Autodesk Inventor part; units mm, degrees
ref_plane "YZ Plane" through (0, 0, 0) normal (1, 0, 0) x (0, 1, 0)
ref_plane "XZ Plane" through (0, 0, 0) normal (0, 1, 0) x (-1, 0, 0)
ref_plane "XY Plane" through (0, 0, 0) normal (0, 0, 1) x (1, 0, 0)
sketch "Sketch1" plane through (0, 0, 0) normal (0, 0, 1) x (1, 0, 0)
  line L0 (0, 0) -> (34, 0)
  line L1 (34, 0) -> (34, 40)
  line L2 (34, 40) -> (0, 40)
  line L3 (0, 40) -> (0, 0)
  line L4 (-10, 30) -> (0, 30)
  line L5 (0, 30) -> (0, 0)
  line L6 (0, 0) -> (-10, 0)
  line L7 (-10, 0) -> (-10, 30)
  line L8 (-10, 30) -> (0, 0) construction
  line L9 (0, 30) -> (-10, 0) construction
  line L10 (44, 30) -> (34, 30)
  line L11 (34, 30) -> (34, 0)
  line L12 (34, 0) -> (44, 0)
  line L13 (44, 0) -> (44, 30)
  line L14 (44, 30) -> (34, 0) construction
  line L15 (34, 30) -> (44, 0) construction
  line L16 (9.5, 32.5) -> (24.5, 32.5)
  line L17 (24.5, 32.5) -> (24.5, 7.5)
  line L18 (24.5, 7.5) -> (9.5, 7.5)
  line L19 (9.5, 7.5) -> (9.5, 32.5)
  line L20 (9.5, 32.5) -> (24.5, 7.5) construction
  line L21 (24.5, 32.5) -> (9.5, 7.5) construction
  point P0 (-5, 15)
  point P1 (39, 15)
  point P2 (0, 20)
  point P3 (0, 15)
  point P4 (34, 30)
  point P5 (0, 30)
  point P6 (17, 20)
  point P7 (17, 40)
  point P8 (34, 20)
  dimension "d0" = 34
  dimension "d1" = 40
  dimension "d2" = 10
  dimension "d3" = 10
  dimension "d4" = 30
  dimension "d5" = 30
  dimension "d8" = 15
  dimension "d9" = 25
extrude "Extrusion1" add sketch "Sketch1" along normal blind 3
properties part number "Frontrail"
The listing builds one solid part. Answer for the finished solid, in the listing's coordinates (mm). A direction names the side the tool comes from. Coordinates: 2 decimals unless noted, no trailing zeros. Write each loop counter-clockwise with the first axis right and the second up, starting at its lowest first coordinate (ties: lowest second). Pieces come first, ordered by that corner, then holes. Notation, with made-up numbers: M -36.5,25 L -28.5,25 A36 ccw -28.5,64 Z; hole C -13,38 d10. An arc over 180 degrees is marked long. Write each question's results on one line, items separated by ' | '.
Item 1: The part is cut by section B-B on z = 1.85. Determine the outline of the cut face in (x, y), and give its area (4 significant figures).
Answer below:
outline: M -10,0 L 44,0 L 44,30 L 34,30 L 34,40 L 0,40 L 0,30 L -10,30 Z; hole M 9.5,7.5 L 24.5,7.5 L 24.5,32.5 L 9.5,32.5 Z | area: 1,585 mm2
Item 2: Consider probe 1 along X at (y, z) = (23, 2.5); probe 2 along Y at (x, z) = (24, 2.75); probe 3 along Y at (x, z) = (38, 2.25). Determine where each line is inside the solid, lowest interval first. Write a range as [from, to].
Answer below:
probe 1: [-10, 9.5], [24.5, 44] | probe 2: [0, 7.5], [32.5, 40] | probe 3: [0, 30]
Item 3: The part is cut by section A-A on y = 9.5. Determine the outline of the cut face in (x, z).
Answer below:
outline: M -10,0 L 9.5,0 L 9.5,3 L -10,3 Z; M 24.5,0 L 44,0 L 44,3 L 24.5,3 Z
Item 4: Which of the six approach directions +Z, -Z, +X, -X, +Y, -Y give full straight-line access (tool end or side, diameter ignored) to faces 4 (the face through (39, 30, 1)), 5 (the face through (24.5, 20, 1)), 6 (the face through (44, 15, 1)), 7 (the face through (17, 40, 1)), 8 (the face through (0, 35, 1))?
Answer below:
face 4: +Z, -Z, +X, +Y | face 5: +Z, -Z | face 6: +Z, -Z, +X, +Y, -Y | face 7: +Z, -Z, +X, -X, +Y | face 8: +Z, -Z, -X, +Y
Item 5: The part is cut by section D-D on x = -6. Determine the outline of the cut face in (y, z), and give its area (3 significant figures).
Answer below:
outline: M 0,0 L 30,0 L 30,3 L 0,3 Z | area: 90.0 mm2
Item 6: The part is cut by section C-C on x = 10.5. Determine the outline of the cut face in (y, z), and give its area (3 significant figures).
Answer below:
outline: M 0,0 L 7.5,0 L 7.5,3 L 0,3 Z; M 32.5,0 L 40,0 L 40,3 L 32.5,3 Z | area: 45.0 mm2
Item 7: For a pull along Y with two mould halves and no side action, classify faces 1 (the face through (17, 7, 0)), 2 (the face through (17, 0, 1)), 3 (the face through (17, 32.5, 1)) as released by +Y, released by -Y, zero draft, split by the parting line, or undercut.
Answer below:
face 1: zero draft | face 2: released by -Y | face 3: undercut
Item 8: Given P1, Ø4, axis at x = 6, y = 11, coming from the -Z side; P2, Ø0.9, axis at y = 35.5, z = 2, coming from the +X side; P3, Ø1.5, axis at x = 41.5, z = 2, coming from the +Y side; P4, Ø4, axis at x = 20.5, y = 11, coming from the +Z side, each flat-ended and moving along its own axis, determine where each tip first touches the part or whether it passes through.
Answer below:
P1: z = 0 | P2: x = 34 | P3: y = 30 | P4: through
